Could you check a few things on this model? Use its own coordinates, in mm. Face numbers are marked on the shaded views. A direction names the side the tool comes from. Round coordinates to 2 decimals unless told otherwise and drop trailing zeros. Loops run counter-clockwise (first coordinate to the right, second up) from the corner with the lowest first, then second, coordinate; pieces in that order, holes last. Notation, with made-up numbers: (57, -4) -> (88, -4) arc R26 ccw to (88, 19) -> close; hole circle Ø6 at (44.5, 16.25). An arc over 180 degrees is marked (long way). Write each question's results on one line, items separated by ' | '. Start each with the question number.
1) Imagine slicing it at B-B, the plane y = 0. List the corners of the cut face in (x, z) for me, plus the area to 3 significant figures.
2) Imagine slicing it at D-D, the plane y = -4.5. List the corners of the cut face in (x, z) for me, plus the area to 4 significant figures.
3) Imagine slicing it at C-C, the plane z = 4.75. List the corners of the cut face in (x, y) for me.
4) Which directions (+Z, -Z, +X, -X, +Y, -Y) give clear straight access to the entire face, cutting with the end or side of a thin tool? Please do the marked faces 1 and 2.
5) If I drill on probe 1 along Z at (x, y) = (1.25, 5.75); probe 2 along X at (y, z) = (-0.25, 3.25); probe 3 along X at (y, z) = (7.5, 2.5), over which ranges is the centre line in solid material (lowest first)?
6) Imagine slicing it at A-A, the plane x = 0. List the corners of the cut face in (y, z) for me.
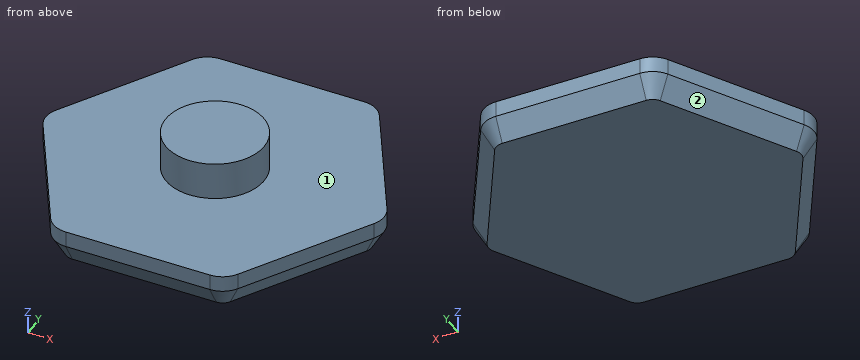
from build123d import *

# Parameters (mm, degrees)
F1_R     = 3.9
F2_DEPTH = 3
F3_R     = 3.9
F4_DEPTH = 6
F5_R     = 2
F6_SIZE2 = 1.7320508076
F6_SIZE  = 1


with BuildPart() as f2:
    # F1 (on face) → F2 (new body)
    with BuildSketch(Plane.XY):
        Polygon((-6.9282032303, -12), (6.9282032303, -12), (13.8564064606, 0), (6.9282032303, 12), (-6.9282032303, 12), (-13.8564064606, 0), align=None)
        Circle(F1_R, mode=Mode.SUBTRACT)
    extrude(amount=F2_DEPTH)

    # F3 (on Top) → F4 (join)
    with BuildSketch(Plane.XY):
        Circle(F3_R)
    extrude(amount=F4_DEPTH)

    # F5
    f5_edges = [f2.edges().sort_by_distance(p)[0] for p in [
        (13.856406, 0, 1.5),
        (6.928203, -12, 1.5),
        (-6.928203, -12, 1.5),
        (-13.856406, 0, 1.5),
        (-6.928203, 12, 1.5),
        (6.928203, 12, 1.5),
    ]]
    fillet(f5_edges, radius=F5_R)

    # F6
    f6_edges = [f2.edges().sort_by_distance(p)[0] for p in [
        (0, -12, 0),
    ]]
    f6_side = f2.faces().sort_by_distance((0, 0, 0))[0]
    chamfer(f6_edges, length=F6_SIZE, length2=F6_SIZE2, reference=f6_side)


solid = f2.part
Checked values:
1) outline: (-13.55, 1.73) -> (-12.55, 0) -> (12.55, 0) -> (13.55, 1.73) -> (13.55, 3) -> (3.9, 3) -> (3.9, 6) -> (-3.9, 6) -> (-3.9, 3) -> (-13.55, 3) -> close | area: 103 mm^2
2) outline: (-11.26, 1.73) -> (-10.1, 0) -> (10.1, 0) -> (11.26, 1.73) -> (11.26, 3) -> (-11.26, 3) -> close | area: 65.55 mm^2
3) outline: circle Ø7.8 at (0, 0)
4) face 1: +Z | face 2: -Z, -X, +Y
5) probe 1: 0 to 3 | probe 2: -3.89 to 3.89 | probe 3: -9.53 to 9.53
6) outline: (-12, 1.73) -> (-11, 0) -> (11, 0) -> (12, 1.73) -> (12, 3) -> (3.9, 3) -> (3.9, 6) -> (-3.9, 6) -> (-3.9, 3) -> (-12, 3) -> close
